from build123d import *

# Parameters (mm, degrees)
F0_W     = 127
F0_H     = 101.6
F1_DEPTH = 38.1
F2_R     = 37.094784
F3_DEPTH = 76.201


with BuildPart() as f1:
    # F0 (on Front) → F1 (new body, symmetric)
    with BuildSketch(Plane.XZ):
        with Locations((-1.06249, -2.622532)):
            Rectangle(F0_W, F0_H)
    extrude(amount=F1_DEPTH, both=True)

    # F2 (on face) → F3 (cut, through all)
    with BuildSketch(Plane.XZ.offset(38.1)):
        Circle(F2_R)
    extrude(amount=-F3_DEPTH, mode=Mode.SUBTRACT)


solid = f1.part
Geometry: final body of the model. Coordinates: model frame, mm. Coordinates: 2 decimals unless noted, no trailing zeros. Order: outer loops, then holes, each group sorted by start corner. A loop starts at its lowest first (then second) coordinate and runs counter-clockwise, first axis right, second up.
(1) Draft query along X for faces 1 (the face through (-8.041, -0.533, -36.213)), 2 (the face through (-64.562, -1, -3)), 3 (the face through (62.438, -1, -3)), 4 (the face through (-2, -1, 48.177)). Return one class per face: pulls with the +X half, pulls with the -X half, needs draft (parallel to the pull), parting line crosses it, or undercut.
(2) Section query C-C (y = 4). Return the cut outline in (x, z), plus the area to 3 significant figures.
(3) Section query A-A (x = 0). Return the cut outline in (y, z).
(4) Section query B-B (z = 0). Return the cut outline in (x, y).
(5) Material intervals for probe 1 along Z at (x, y) = (0, 0); probe 2 along X at (y, z) = (-14, -4.5); probe 3 along X at (y, z) = (-21, 16.5), sorted ascending.
Solution:
1. face 1: undercut
1. face 2: pulls with the -X half
1. face 3: pulls with the +X half
1. face 4: needs draft
2. outline: (-64.56, -53.42) - (62.44, -53.42) - (62.44, 48.18) - (-64.56, 48.18) - close; hole circle Ø74.19 at (0, 0)
2. area: 8,580 mm2
3. outline: (-38.1, -53.42) - (38.1, -53.42) - (38.1, -37.09) - (-38.1, -37.09) - close; (-38.1, 37.09) - (38.1, 37.09) - (38.1, 48.18) - (-38.1, 48.18) - close
4. outline: (-64.56, -38.1) - (-37.09, -38.1) - (-37.09, 38.1) - (-64.56, 38.1) - close; (37.09, -38.1) - (62.44, -38.1) - (62.44, 38.1) - (37.09, 38.1) - close
5. probe 1: z = -53.42 to -37.09, 37.09 to 48.18
5. probe 2: x = -64.56 to -36.82, 36.82 to 62.44
5. probe 3: x = -64.56 to -33.22, 33.22 to 62.44
